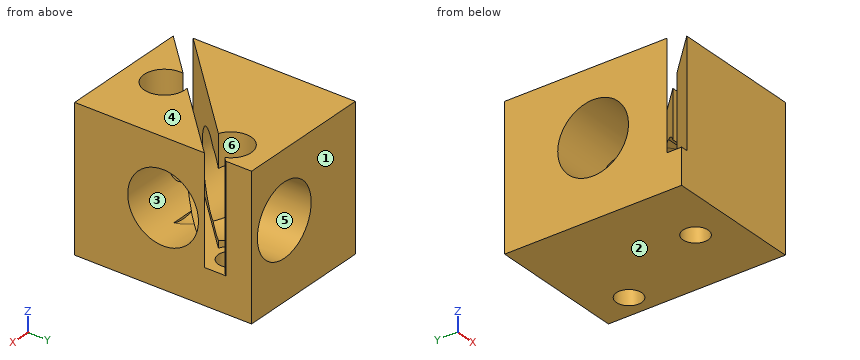
```python
from build123d import *

# Parameters (mm, degrees)
SKETCH_W        = 27
SKETCH_H        = 35
SKETCH_R        = 2.5
PAD_DEPTH       = 28
POCKET_DEPTH    = 21
SKETCH002_R     = 7
POCKET001_DEPTH = 20
SKETCH003_R     = 7
POCKET002_DEPTH = 27.001
SKETCH004_R     = 4
POCKET003_DEPTH = 21


with BuildPart() as part:
    # Sketch → Pad (new body)
    with BuildSketch(Plane.XY):
        with Locations((3.5, 0)):
            Rectangle(SKETCH_W, SKETCH_H)
        with Locations((3.5, -10)):
            Circle(SKETCH_R, mode=Mode.SUBTRACT)
        with Locations((12.5, 10)):
            Circle(SKETCH_R, mode=Mode.SUBTRACT)
    extrude(amount=PAD_DEPTH)

    # Sketch001 (on Face1 of CopyCut001) → Pocket (cut)
    with BuildSketch(Plane.XY.offset(28)):
        Polygon((17, 12.392641), (-10, -14.607359), (-10, -18.85), (17, 8.15), align=None)
    extrude(amount=-POCKET_DEPTH, mode=Mode.SUBTRACT)

    # Sketch002 (on Face1 of Pocket) → Pocket001 (cut)
    with BuildSketch(Plane(origin=(0, 17.5, 0), x_dir=(-1, 0, 0), z_dir=(0, 1, 0))):
        with Locations((-8.5, 15)):
            Circle(SKETCH002_R)
    extrude(amount=-POCKET001_DEPTH, mode=Mode.SUBTRACT)

    # Sketch003 (on Face5 of Pocket001) → Pocket002 (cut, through all)
    with BuildSketch(Plane.YZ.offset(17)):
        with Locations((0, 15)):
            Circle(SKETCH003_R)
    extrude(amount=-POCKET002_DEPTH, mode=Mode.SUBTRACT)

    # Sketch004 (on Sketch) → Pocket003 (cut)
    with BuildSketch(Plane(origin=(8, 0, 28), x_dir=(0.911922, -0.410365, 0), z_dir=(0, 0, 1))):
        with Locations((0, 10.965856)):
            Circle(SKETCH004_R)
        with Locations((0, -10.965856)):
            Circle(SKETCH004_R)
    extrude(amount=-POCKET003_DEPTH, mode=Mode.SUBTRACT)


solid = part.part
```
Can you work these out from the model? Positions are in its coordinate system, mm. Face numbers are marked on the shaded views. A direction names the side the tool comes from. Coordinates: 2 decimals unless noted, no trailing zeros. Loops run counter-clockwise (first coordinate to the right, second up) from the corner with the lowest first, then second, coordinate; pieces in that order, holes last. Notation, with made-up numbers: (-6, -16) -> (22, -16) arc R25 cw to (22, 4) -> close; hole circle Ø9 at (59.25, -24.75). An arc over 180 degrees is marked (long way). Answer as a JSON object with one key per item and string values.
1) For P1, Ø11, axis at x = 8.5, z = 15, coming from the +Y side; P2, Ø3, axis at x = 4, z = 18, coming from the +Y side; P3, Ø6.5, axis at x = 3.5, y = -10, coming from the +Z side, each with a flat end and sliding along its axis, tell me the tip position at first contact or that it passes through.
Results:
{"P1": "stops at y = -4.33", "P2": "stops at y = -5.36", "P3": "stops at z = 7"}
2) Imagine slicing it at D-D (y = 1). Please give me the cut outline in (x, z).
Results:
{"outline": "(-10, 0) -> (17, 0) -> (17, 8.07) -> (9.85, 8.07) -> (9.85, 7) -> (5.61, 7) -> (5.61, 8.07) -> (-10, 8.07) -> close; (-10, 21.93) -> (5.61, 21.93) -> (5.61, 28) -> (-10, 28) -> close; (9.85, 21.93) -> (17, 21.93) -> (17, 28) -> (9.85, 28) -> close"}
3) For the marked faces 4, 5 and 6, which set-ups out of +Z, -Z, +X, -X, +Y, -Y let a thin tool reach every point of the face, with its end or its side?
Results:
{"face 4": "+Z, +X, -X, +Y, -Y", "face 5": "+Y", "face 6": "+Z"}
4) Imagine slicing it at A-A (y = 10). Please give me the cut outline in (x, z), then the cut area to 3 significant figures.
Results:
{"outline": "(-10, 0) -> (10, 0) -> (10, 7) -> (8.5, 7) -> (8.5, 8) arc R7 cw to (8.5, 22) -> (8.5, 28) -> (-10, 28) -> close; (15, 0) -> (17, 0) -> (17, 7) -> (15, 7) -> close", "area": "466 mm^2"}
5) Imagine slicing it at C-C (x = 3.5). Please give me the cut outline in (y, z), then the cut area to 3 significant figures.
Results:
{"outline": "(-17.5, 0) -> (-12.5, 0) -> (-12.5, 7) -> (-14, 7) -> (-14, 28) -> (-17.5, 28) -> close; (-7.5, 0) -> (17.5, 0) -> (17.5, 10.1) -> (5, 10.1) arc R7 cw to (-1.11, 8.09) -> (-1.11, 7) -> (-5.35, 7) -> (-5.35, 10.49) arc R7 cw to (-6, 11.39) -> (-6, 7) -> (-7.5, 7) -> close; (-6, 18.61) arc R7 cw to (-5.35, 19.51) -> (-5.35, 28) -> (-6, 28) -> close; (-1.11, 21.91) arc R7 cw to (5, 19.9) -> (17.5, 19.9) -> (17.5, 28) -> (-1.11, 28) -> close", "area": "481 mm^2"}
6) Thinking about a two-plate mould opening in Y: for the marked faces 1, 2 and 3, which applies, pulls with the +Y half, pulls with the -Y half, needs draft (parallel to the pull), parting line crosses it, or undercut?
Results:
{"face 1": "pulls with the +Y half", "face 2": "needs draft", "face 3": "undercut"}
7) Imagine slicing it at B-B (z = 21). Please give me the cut outline in (x, y).
Results:
{"outline": "(-10, -14.61) -> (1, -3.61) -> (-10, -3.61) -> close; (-10, 3.61) -> (4.89, 3.61) -> (4.89, 17.5) -> (-10, 17.5) -> close; (-8.65, -17.5) -> (17, -17.5) -> (17, -3.61) -> (5.24, -3.61) -> (2.79, -6.06) arc R4 cw (long way) to (-0.44, -9.29) -> close; (12.11, 13.98) arc R4 cw to (16.18, 11.57) -> (17, 12.39) -> (17, 17.5) -> (12.11, 17.5) -> close; (12.46, 3.61) -> (17, 3.61) -> (17, 8.15) -> close"}
8) If I drill on line 1 (Y direction, x = 12.5, z = 3.5); line 2 (Z direction, x = -3.75, y = 0); line 3 (X direction, y = -10, z = 5), over which ranges is the centre line in solid material (lowest first)?
Results:
{"line 1": "y = -17.5 to 7.5, 12.5 to 17.5", "line 2": "z = 0 to 8, 22 to 28", "line 3": "x = -10 to 1, 6 to 17"}
